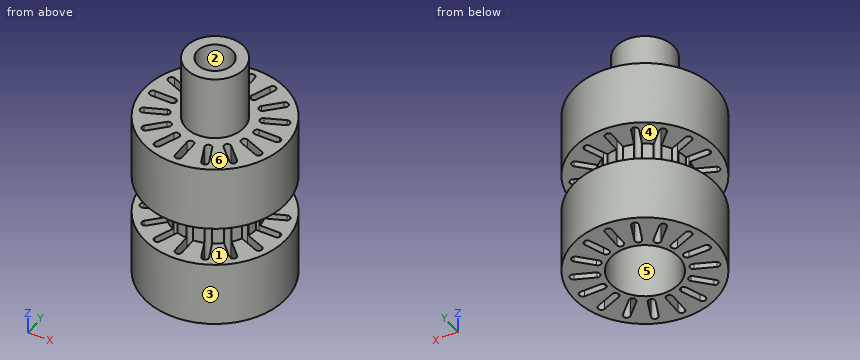
from build123d import *

# Parameters (mm, degrees)
CUT_EXTRUDE1_DEPTH = 86


with BuildPart() as part:
    # Sketch1 → Revolve1 (revolve)
    with BuildSketch(Plane(origin=(0, 0, 0), x_dir=(0, 0, -1), z_dir=(1, 0, 0))):
        Polygon((-15, 0), (15, 0), (3.6, 0), align=None)
        Polygon((-15, 5.1), (-15, 12.5), (-3.5, 12.5), (-3.5, 7.5), (3.5, 7.5), (3.5, 12.5), (15, 12.5), (15, 6), (3.6, 6), (3.6, 3.1), (-15, 3.1), (-26.4, 3.1), (-26.4, 5.1), align=None)
    revolve(axis=Axis((0, 0, 15), (0, 0, -1)))

    # Sketch2 → Cut-Extrude1 (cut)
    with BuildSketch(Plane(origin=(0, 0, -15), x_dir=(-1, 0, 0), z_dir=(0, 0, -1))):
        with BuildLine():
            Line((0.59414275, 10.8), (0.59414275, 7.3))
            ThreePointArc((0.59414275, 7.3), (0, 6.70585725), (-0.59414275, 7.3))
            Line((-0.59414275, 7.3), (-0.59414275, 10.8))
            ThreePointArc((-0.59414275, 10.8), (0, 11.39414275), (0.59414275, 10.8))
        make_face()
        with BuildLine():
            Line((3.584064744, 10.205267538), (2.24467273, 6.971689174))
            ThreePointArc((2.24467273, 6.971689174), (2.566220469, 6.195404261), (3.342505382, 6.516952001))
            Line((3.342505382, 6.516952001), (4.681897395, 9.750530364))
            ThreePointArc((4.681897395, 9.750530364), (4.360349656, 10.526815277), (3.584064744, 10.205267538))
        make_face()
        with BuildLine():
            Line((7.216630869, 8.056875604), (4.741757135, 5.58200187))
            ThreePointArc((4.741757135, 5.58200187), (4.741757135, 4.741757135), (5.58200187, 4.741757135))
            Line((5.58200187, 4.741757135), (8.056875604, 7.216630869))
            ThreePointArc((8.056875604, 7.216630869), (8.056875604, 8.056875604), (7.216630869, 8.056875604))
        make_face()
        with BuildLine():
            Line((9.750530364, 4.681897395), (6.516952001, 3.342505382))
            ThreePointArc((6.516952001, 3.342505382), (6.195404261, 2.566220469), (6.971689174, 2.24467273))
            Line((6.971689174, 2.24467273), (10.205267538, 3.584064744))
            ThreePointArc((10.205267538, 3.584064744), (10.526815277, 4.360349656), (9.750530364, 4.681897395))
        make_face()
        with BuildLine():
            Line((10.8, 0.59414275), (7.3, 0.59414275))
            ThreePointArc((7.3, 0.59414275), (6.70585725, 0), (7.3, -0.59414275))
            Line((7.3, -0.59414275), (10.8, -0.59414275))
            ThreePointArc((10.8, -0.59414275), (11.39414275, 0), (10.8, 0.59414275))
        make_face()
        with BuildLine():
            Line((10.205267538, -3.584064744), (6.971689174, -2.24467273))
            ThreePointArc((6.971689174, -2.24467273), (6.195404261, -2.566220469), (6.516952001, -3.342505382))
            Line((6.516952001, -3.342505382), (9.750530364, -4.681897395))
            ThreePointArc((9.750530364, -4.681897395), (10.526815277, -4.360349656), (10.205267538, -3.584064744))
        make_face()
        with BuildLine():
            Line((8.056875604, -7.216630869), (5.58200187, -4.741757135))
            ThreePointArc((5.58200187, -4.741757135), (4.741757135, -4.741757135), (4.741757135, -5.58200187))
            Line((4.741757135, -5.58200187), (7.216630869, -8.056875604))
            ThreePointArc((7.216630869, -8.056875604), (8.056875604, -8.056875604), (8.056875604, -7.216630869))
        make_face()
        with BuildLine():
            Line((4.681897395, -9.750530364), (3.342505382, -6.516952001))
            ThreePointArc((3.342505382, -6.516952001), (2.566220469, -6.195404261), (2.24467273, -6.971689174))
            Line((2.24467273, -6.971689174), (3.584064744, -10.205267538))
            ThreePointArc((3.584064744, -10.205267538), (4.360349656, -10.526815277), (4.681897395, -9.750530364))
        make_face()
        with BuildLine():
            Line((0.59414275, -10.8), (0.59414275, -7.3))
            ThreePointArc((0.59414275, -7.3), (0, -6.70585725), (-0.59414275, -7.3))
            Line((-0.59414275, -7.3), (-0.59414275, -10.8))
            ThreePointArc((-0.59414275, -10.8), (0, -11.39414275), (0.59414275, -10.8))
        make_face()
        with BuildLine():
            Line((-3.584064744, -10.205267538), (-2.24467273, -6.971689174))
            ThreePointArc((-2.24467273, -6.971689174), (-2.566220469, -6.195404261), (-3.342505382, -6.516952001))
            Line((-3.342505382, -6.516952001), (-4.681897395, -9.750530364))
            ThreePointArc((-4.681897395, -9.750530364), (-4.360349656, -10.526815277), (-3.584064744, -10.205267538))
        make_face()
        with BuildLine():
            Line((-7.216630869, -8.056875604), (-4.741757135, -5.58200187))
            ThreePointArc((-4.741757135, -5.58200187), (-4.741757135, -4.741757135), (-5.58200187, -4.741757135))
            Line((-5.58200187, -4.741757135), (-8.056875604, -7.216630869))
            ThreePointArc((-8.056875604, -7.216630869), (-8.056875604, -8.056875604), (-7.216630869, -8.056875604))
        make_face()
        with BuildLine():
            Line((-9.750530364, -4.681897395), (-6.516952001, -3.342505382))
            ThreePointArc((-6.516952001, -3.342505382), (-6.195404261, -2.566220469), (-6.971689174, -2.24467273))
            Line((-6.971689174, -2.24467273), (-10.205267538, -3.584064744))
            ThreePointArc((-10.205267538, -3.584064744), (-10.526815277, -4.360349656), (-9.750530364, -4.681897395))
        make_face()
        with BuildLine():
            Line((-10.8, -0.59414275), (-7.3, -0.59414275))
            ThreePointArc((-7.3, -0.59414275), (-6.70585725, 0), (-7.3, 0.59414275))
            Line((-7.3, 0.59414275), (-10.8, 0.59414275))
            ThreePointArc((-10.8, 0.59414275), (-11.39414275, 0), (-10.8, -0.59414275))
        make_face()
        with BuildLine():
            Line((-10.205267538, 3.584064744), (-6.971689174, 2.24467273))
            ThreePointArc((-6.971689174, 2.24467273), (-6.195404261, 2.566220469), (-6.516952001, 3.342505382))
            Line((-6.516952001, 3.342505382), (-9.750530364, 4.681897395))
            ThreePointArc((-9.750530364, 4.681897395), (-10.526815277, 4.360349656), (-10.205267538, 3.584064744))
        make_face()
        with BuildLine():
            Line((-8.056875604, 7.216630869), (-5.58200187, 4.741757135))
            ThreePointArc((-5.58200187, 4.741757135), (-4.741757135, 4.741757135), (-4.741757135, 5.58200187))
            Line((-4.741757135, 5.58200187), (-7.216630869, 8.056875604))
            ThreePointArc((-7.216630869, 8.056875604), (-8.056875604, 8.056875604), (-8.056875604, 7.216630869))
        make_face()
        with BuildLine():
            Line((-4.681897395, 9.750530364), (-3.342505382, 6.516952001))
            ThreePointArc((-3.342505382, 6.516952001), (-2.566220469, 6.195404261), (-2.24467273, 6.971689174))
            Line((-2.24467273, 6.971689174), (-3.584064744, 10.205267538))
            ThreePointArc((-3.584064744, 10.205267538), (-4.360349656, 10.526815277), (-4.681897395, 9.750530364))
        make_face()
    extrude(amount=-CUT_EXTRUDE1_DEPTH, mode=Mode.SUBTRACT)


solid = part.part
Geometry check sheet. Reference: the model listing, model coordinates, mm. Face numbers are marked on the shaded views. A direction names the side the tool comes from. Round coordinates to 2 decimals unless told otherwise and drop trailing zeros. Loops run counter-clockwise (first coordinate to the right, second up) from the corner with the lowest first, then second, coordinate; pieces in that order, holes last. Notation, with made-up numbers: (-28, 32.5) -> (-22, 32.5) arc R11 ccw to (-22, 49.5) -> close; hole circle Ø1 at (20, -22). An arc over 180 degrees is marked (long way). Answer as a JSON object with one key per item and string values. Group by question number.
Item 1: Thickness scan on line 1 along X through (y, z) = (0, 7.5); line 2 along X through (y, z) = (0, -9); line 3 along X through (y, z) = (0, 20). Record the ranges inside material, lowest first.
Item 2: Depth check by flat-ended pin: pin 1 Ø6 at (x, y) = (2.5, -2) entering from -Z; pin 2 Ø3 at (x, z) = (-7, -7) entering from -Y (3 decimals); pin 3 Ø3 at (y, z) = (-9.5, 4) entering from -X; pin 4 Ø4 at (y, z) = (-8.5, 6) entering from +X. Enter the tip coordinate at first touch or a pass-through.
Item 3: Cross-section at A-A, the plane x = 0. Count the separate pieces of the cut face and the enclosed holes in it, plus the area to 3 significant figures.
Item 4: Cross-section at C-C, the plane z = 15.5. Record the cut outline in (x, y).
Item 5: Release check for a two-part mould opening along X. For the marked faces 1, 2 and 3 record: pulls with the +X half, pulls with the -X half, needs draft (parallel to the pull), parting line crosses it, or undercut.
Item 6: Set-up check for the marked faces 4, 5 and 6: record each of +Z, -Z, +X, -X, +Y, -Y from which the full face is reachable in a straight line by a thin tool's end or side.
Determined:
{
 "1": {"line 1": "x = -12.5 to -11.39, -6.71 to -3.1, 3.1 to 6.71, 11.39 to 12.5", "line 2": "x = -12.5 to -11.39, -6.71 to -6, 6 to 6.71, 11.39 to 12.5", "line 3": "x = -5.1 to -3.1, 3.1 to 5.1"},
 "2": {"pin 1": "stops at z = -15", "pin 2": "stops at y = -11.225", "pin 3": "stops at x = -9.6", "pin 4": "stops at x = 10.68"},
 "3": {"separate pieces": "6", "enclosed holes": "0", "area": "247 mm²"},
 "4": {"outline": "circle Ø10.2 at (0, 0); hole circle Ø6.2 at (0, 0)"},
 "5": {"face 1": "needs draft", "face 2": "undercut", "face 3": "parting line crosses it"},
 "6": {"face 4": "none", "face 5": "-Z", "face 6": "+Z"}
}
